Read the model definition and answer for the solid it produces. Units are mm, in the model's axes. A direction names the side the tool comes from. Round coordinates to 2 decimals unless told otherwise and drop trailing zeros. Order: outer loops, then holes, each group sorted by start corner. A loop starts at its lowest first (then second) coordinate and runs counter-clockwise, first axis right, second up. Notation, with made-up numbers: (-23.75, 55) - (21.25, 55) arc R17 cw to (21.25, 73) - close; hole circle Ø2 at (82, 83). An arc over 180 degrees is marked (long way). Put each result on its own line as item: value. Start each with the question number.
Q1. Section B-B on x = 4 is taken. State how many separate pieces and enclosed holes the cut face has, then the cut area to 3 significant figures.
Q2. Which of the six approach directions +Z, -Z, +X, -X, +Y, -Y give full straight-line access (tool end or side, diameter ignored) to faces 1 (the face through (5, -9, 0)), 2 (the face through (10, -24, -9)), 3 (the face through (5, -39, 7.87)), 4 (the face through (5, -34, -35.67))?
Q3. Find the intervals of material crossed by line 1 along Y through (x, z) = (2.25, -13.8) (3 decimals); line 2 along Y through (x, z) = (3.5, 27.5); line 3 along Z through (x, y) = (0.5, -42.5), in increasing order. Write a range as from..to.
Q4. For a pull along Z with two mould halves and no side action, classify faces 5 (the face through (4.93, -48.059, 9.073)), 6 (the face through (5, -9, -17.8)), 7 (the face through (5.07, -5.25, -2.37)), 8 (the face through (5, -49.2, 20)) as pulls with the +Z half, pulls with the -Z half, needs draft (parallel to the pull), parting line crosses it, or undercut.
Q5. Section A-A on z = -40 is taken. Give the vertices of the cut face in (x, y).
Q6. Each of these flat-tipped pins is pushed along its axis until it touches: pin 1 Ø3 at (x, z) = (3, -43.5) entering from +Y; pin 2 Ø3 at (x, y) = (4, -35) entering from -Z; pin 3 Ø5 at (x, y) = (5.5, -37) entering from +Z; pin 4 Ø1 at (x, z) = (4.5, -9.5) entering from -Y. Where does it stop, or does it pass through?
Q7. Section C-C on z = 7 is taken. Give the vertices of the cut face in (x, y).
from build123d import *

# Parameters (mm, degrees)
BOSS_EXTRUDE1_DEPTH = 10
SKETCH3_R           = 2.055
CUT_EXTRUDE1_DEPTH  = 11
BOSS_EXTRUDE2_DEPTH = 10
FILLET1_R           = 4
FILLET2_R           = 4


with BuildPart() as part:
    # Sketch1 → Boss-Extrude1 (new body)
    with BuildSketch(Plane(origin=(0, 0, 0), x_dir=(0, 0, -1), z_dir=(1, 0, 0))):
        Polygon((17.8, -18.8), (50, -18.8), (50, -28.8), (-32.2, -28.8), (-32.2, -18.8), (0, -18.8), (0, 0), (17.8, 0), align=None)
    extrude(amount=BOSS_EXTRUDE1_DEPTH)

    # Sketch3 → Cut-Extrude1 (cut, through all)
    with BuildSketch(Plane(origin=(10, 0, 0), x_dir=(0, 0, -1), z_dir=(1, 0, 0))):
        with Locations((4, -4)):
            Circle(SKETCH3_R)
        with Locations((13.8, -4)):
            Circle(SKETCH3_R)
    extrude(amount=-CUT_EXTRUDE1_DEPTH, mode=Mode.SUBTRACT)

    # Sketch4 → Boss-Extrude2 (add)
    with BuildSketch(Plane(origin=(10, 0, 0), x_dir=(0, 0, -1), z_dir=(1, 0, 0))):
        Polygon((-17.87, -28.8), (-17.87, -39.2), (-32.2, -39.2), (-32.2, -49.2), (-7.87, -49.2), (-7.87, -28.8), align=None)
        Polygon((35.67, -28.8), (25.67, -28.8), (25.67, -49.2), (50, -49.2), (50, -39.2), (35.67, -39.2), align=None)
    extrude(amount=-BOSS_EXTRUDE2_DEPTH)

    # Fillet1
    fillet1_edges = [part.edges().sort_by_distance(p)[0] for p in [
        (5, 0, 0),
        (5, 0, -17.8),
    ]]
    fillet(fillet1_edges, radius=FILLET1_R)

    # Fillet2
    fillet2_edges = [part.edges().sort_by_distance(p)[0] for p in [
        (5, -18.8, -17.8),
        (5, -18.8, -50),
        (5, -18.8, 32.2),
        (5, -18.8, 0),
        (5, -49.2, 32.2),
        (5, -49.2, 7.87),
        (5, -28.8, 7.87),
        (5, -28.8, -25.67),
        (5, -49.2, -25.67),
        (5, -49.2, -50),
    ]]
    fillet(fillet2_edges, radius=FILLET2_R)


solid = part.part
Findings:
1. separate pieces: 1
1. enclosed holes: 2
1. area: 1,810 mm2
2. face 1: +Z, +X, -X, +Y
2. face 2: +Z, -Z, +X, +Y, -Y
2. face 3: +X, -X, -Y
2. face 4: -Z, +X, -X
3. line 1: -28.8..-6.055, -1.945..0
3. line 2: -49.2..-39.2, -28.8..-18.8
3. line 3: -50..-25.67, 7.87..32.2
4. face 5: undercut
4. face 6: pulls with the -Z half
4. face 7: undercut
4. face 8: needs draft
5. outline: (0, -49.2) - (10, -49.2) - (10, -39.2) - (0, -39.2) - close; (0, -28.8) - (10, -28.8) - (10, -18.8) - (0, -18.8) - close
6. pin 1: y = -18.8
6. pin 2: z = -35.67
6. pin 3: z = 32.2
6. pin 4: y = -28.8
7. outline: (0, -30.31) - (10, -30.31) - (10, -18.8) - (0, -18.8) - close
